Model file for the job. Use its own axes, mm. Round coordinates to 2 decimals unless told otherwise and drop trailing zeros. Loops run counter-clockwise (first coordinate to the right, second up) from the corner with the lowest first, then second, coordinate; pieces in that order, holes last. Notation, with made-up numbers: (69.5, 16) - (111.5, 16) arc R28 ccw to (111.5, 51) - close; hole circle Ø4 at (21, -11.5). An arc over 180 degrees is marked (long way). Use one line per item in the form item = value.
from build123d import *

# Parameters (mm, degrees)
F1_DEPTH = 3
F2_DEPTH = 2.5
F3_D     = 28
F3_DEPTH = 50.5
F3_TIP   = 8.4120486664
F4_D     = 28
F4_DEPTH = 50.5
F4_TIP   = 8.4120486664
F5_D     = 5.5
F5_DEPTH = 14.4
F5_TIP   = 1.6523667023


with BuildPart() as f1:
    # F0 (on Top) → F1 (new body)
    with BuildSketch(Plane.XY):
        with BuildLine():
            ThreePointArc((152.5413805678, -71.0417273613), (151.062304835, -74.5502561039), (147.5415546881, -76))
            Line((147.5415546881, -76), (152.5, -76))
            Line((152.5, -76), (152.5413805678, -71.0417273613))
        make_face()
    extrude(amount=F1_DEPTH)

    # F0 (on Top) → F2 (join)
    with BuildSketch(Plane.XY):
        with BuildLine():
            ThreePointArc((-152.5413805678, -71.0417273613), (-151.062304835, -74.5502561039), (-147.5415546881, -76))
            Line((-147.5415546881, -76), (147.5415546881, -76))
            ThreePointArc((147.5415546881, -76), (151.062304835, -74.5502561039), (152.5413805678, -71.0417273613))
            Line((152.5413805678, -71.0417273613), (152.7503728867, -46))
            Line((152.7503728867, -46), (167.5, -46))
            ThreePointArc((167.5, -46), (171.0355339059, -44.5355339059), (172.5, -41))
            Line((172.5, -41), (172.5, 41))
            ThreePointArc((172.5, 41), (171.0355339059, 44.5355339059), (167.5, 46))
            Line((167.5, 46), (152.7503728867, 46))
            Line((152.7503728867, 46), (152.5413805678, 71.0417273613))
            ThreePointArc((152.5413805678, 71.0417273613), (151.062304835, 74.5502561039), (147.5415546881, 76))
            Line((147.5415546881, 76), (-147.5415546881, 76))
            ThreePointArc((-147.5415546881, 76), (-151.062304835, 74.5502561039), (-152.5413805678, 71.0417273613))
            Line((-152.5413805678, 71.0417273613), (-152.7503728867, 46))
            Line((-152.7503728867, 46), (-167.5, 46))
            ThreePointArc((-167.5, 46), (-171.0355339059, 44.5355339059), (-172.5, 41))
            Line((-172.5, 41), (-172.5, -41))
            ThreePointArc((-172.5, -41), (-171.0355339059, -44.5355339059), (-167.5, -46))
            Line((-167.5, -46), (-152.7503728867, -46))
            Line((-152.7503728867, -46), (-152.5413805678, -71.0417273613))
        make_face()
    extrude(amount=F2_DEPTH)

    # F3
    with Locations(Plane(origin=(0, 0, 0), x_dir=(1, 0, 0), z_dir=(0, 0, -1))):
        with Locations((0, -76)):
            Hole(F3_D / 2, depth=F3_DEPTH)
            with Locations((0, 0, -(F3_DEPTH + F3_TIP / 2))):  # 118° drill point
                Cone(0, F3_D / 2, F3_TIP, mode=Mode.SUBTRACT)

    # F4
    with Locations(Plane(origin=(0, 0, 0), x_dir=(1, 0, 0), z_dir=(0, 0, -1))):
        with Locations((0, 76)):
            Hole(F4_D / 2, depth=F4_DEPTH)
            with Locations((0, 0, -(F4_DEPTH + F4_TIP / 2))):  # 118° drill point
                Cone(0, F4_D / 2, F4_TIP, mode=Mode.SUBTRACT)

    # F5
    with Locations(Plane(origin=(0, 0, 0), x_dir=(1, 0, 0), z_dir=(0, 0, -1))):
        with Locations((-115, 36), (-115, -36), (115, -36), (115, 36)):
            Hole(F5_D / 2, depth=F5_DEPTH)
            with Locations((0, 0, -(F5_DEPTH + F5_TIP / 2))):  # 118° drill point
                Cone(0, F5_D / 2, F5_TIP, mode=Mode.SUBTRACT)


solid = f1.part
1. Cut at B-B, the plane x = 104.5. Give the cut face in (y, z).
Geometry check:
outline = (-76, 0) - (76, 0) - (76, 2.5) - (-76, 2.5) - close
2. Cut at A-A, the plane z = 0.9. Give the cut face in (x, y), plus the area to 3 significant figures.
Geometry check:
outline = (-172.5, -41) arc R5 ccw to (-167.5, -46) - (-152.75, -46) - (-152.54, -71.04) arc R5 ccw to (-147.54, -76) - (-14, -76) arc R14 cw to (14, -76) - (152.5, -76) - (152.75, -46) - (167.5, -46) arc R5 ccw to (172.5, -41) - (172.5, 41) arc R5 ccw to (167.5, 46) - (152.75, 46) - (152.54, 71.04) arc R5 ccw to (147.54, 76) - (14, 76) arc R14 cw to (-14, 76) - (-147.54, 76) arc R5 ccw to (-152.54, 71.04) - (-152.75, 46) - (-167.5, 46) arc R5 ccw to (-172.5, 41) - close; hole circle Ø5.5 at (-115, -36); hole circle Ø5.5 at (-115, 36); hole circle Ø5.5 at (115, -36); hole circle Ø5.5 at (115, 36)
area = 49,300 mm^2
3. Cut at C-C, the plane y = -9. Give the cut face in (x, z), plus the area to 4 significant figures.
Geometry check:
outline = (-172.5, 0) - (172.5, 0) - (172.5, 2.5) - (-172.5, 2.5) - close
area = 862.5 mm^2
4. Pull direction X, two halves, no side cores. Call faces 1 (the flat face through (-2, 1, 0)), 2 (the cylindrical face through (0, -62, 1)): +X half, -X half, draft (parallel to the pull), parting line (faces both ways), or undercut.
Geometry check:
face_1 = draft
face_2 = undercut
5. Wall check: probe 1 along X at (y, z) = (-36, 1.9); probe 2 along Z at (x, y) = (-85, 17.5); probe 3 along Y at (x, z) = (154.5, 2.45). Give the ranges that are in metal, low to high.
Geometry check:
probe_1 = -172.5 to -117.75, -112.25 to 112.25, 117.75 to 172.5
probe_2 = 0 to 2.5
probe_3 = -46 to 46
6. Flat gauge pins, fed straight in: pin 1 (7 mm diameter, centred on x = 115, y = -36, fed in from +Z); pin 2 (0.8 mm diameter, centred on x = 163, z = 1, fed in from -Y); pin 3 (3.5 mm diameter, centred on x = -115, y = -36, fed in from -Z). Where does each tip first touch, or does it go through?
Geometry check:
pin_1 = 2.5
pin_2 = -46
pin_3 = through
